```python
from build123d import *

# Parameters (mm, degrees)
SKETCH1_R           = 4.826
BOSS_EXTRUDE1_DEPTH = 9.652
SKETCH2_W           = 57.404
SKETCH2_H           = 3.048
CUT_EXTRUDE1_DEPTH  = 98.666302935
SKETCH5_W           = 60.452
SKETCH5_H           = 47.752
BOSS_EXTRUDE2_DEPTH = 7.874
FILLET1_R           = 7.874
SKETCH7_R           = 3.937
CUT_EXTRUDE2_DEPTH  = 7.874
RIB1_REACH          = 137.874
SKETCH11_WALL_W     = 341.312489082
SKETCH11_WALL_H     = 7.874


with BuildPart() as part:
    # Sketch1 → Boss-Extrude1 (new body)
    with BuildSketch(Plane(origin=(0, 0, 0), x_dir=(1, 0, 0), z_dir=(0, 1, 0))):
        with BuildLine():
            Line((-25.4, 60.325), (25.4, 60.325))
            ThreePointArc((25.4, 60.325), (34.380256121, 56.605256121), (38.1, 47.625))
            Line((38.1, 47.625), (38.1, -47.625))
            ThreePointArc((38.1, -47.625), (34.380256121, -56.605256121), (25.4, -60.325))
            Line((25.4, -60.325), (-25.4, -60.325))
            ThreePointArc((-25.4, -60.325), (-34.380256121, -56.605256121), (-38.1, -47.625))
            Line((-38.1, -47.625), (-38.1, 47.625))
            ThreePointArc((-38.1, 47.625), (-34.380256121, 56.605256121), (-25.4, 60.325))
        make_face()
        with Locations(Location((-25.4, -47.625, 0), (0, 0, 270))):
            Circle(SKETCH1_R, mode=Mode.SUBTRACT)
        with Locations(Location((25.4, -47.625, 0), (0, 0, 270))):
            Circle(SKETCH1_R, mode=Mode.SUBTRACT)
        with Locations(Location((25.4, 47.625, 0), (0, 0, 270))):
            Circle(SKETCH1_R, mode=Mode.SUBTRACT)
        with Locations(Location((-25.4, 47.625, 0), (0, 0, 270))):
            Circle(SKETCH1_R, mode=Mode.SUBTRACT)
    extrude(amount=BOSS_EXTRUDE1_DEPTH)

    # Sketch2 → Cut-Extrude1 (cut, through all)
    with BuildSketch(Plane.ZY.offset(38.1)):
        Rectangle(SKETCH2_W, SKETCH2_H)
    extrude(amount=-CUT_EXTRUDE1_DEPTH, mode=Mode.SUBTRACT)



with BuildPart() as body_2:
    # Sketch5 → Boss-Extrude2 (new body)
    with BuildSketch(Plane(origin=(-42.960508789, 74.409783942, 0), x_dir=(0.8660254037844399, 0.49999999999999795, 0), z_dir=(0.4999999999999979, -0.8660254037844398, 0))):
        with Locations((35.838432116, 0)):
            Rectangle(SKETCH5_W, SKETCH5_H)
    extrude(amount=-BOSS_EXTRUDE2_DEPTH)

    # Fillet1
    fillet1_edges = [body_2.edges().sort_by_distance(p)[0] for p in [
        (-40.0685, 80.625542015, 23.876),
        (12.28446771, 110.851542015, 23.876),
        (12.28446771, 110.851542015, -23.876),
        (-40.0685, 80.625542015, -23.876),
    ]]
    fillet(fillet1_edges, radius=FILLET1_R)

    # Sketch7 → Cut-Extrude2 (cut)
    with BuildSketch(Plane(origin=(-46.897508789, 81.228867971, 0), x_dir=(0.8660254037844398, 0.49999999999999806, 0), z_dir=(-0.499999999999998, 0.8660254037844397, 0))):
        with Locations(Location((13.486432116, 16.002, 0), (0, 0, 180))):
            Circle(SKETCH7_R)
        with Locations(Location((13.486432116, -16.002, 0), (0, 0, 180))):
            Circle(SKETCH7_R)
        with Locations(Location((58.190432116, -16.002, 0), (0, 0, 180))):
            Circle(SKETCH7_R)
        with Locations(Location((58.190432116, 16.002, 0), (0, 0, 180))):
            Circle(SKETCH7_R)
    extrude(amount=-CUT_EXTRUDE2_DEPTH, mode=Mode.SUBTRACT)


with BuildPart() as part_1:
    add(part.part)

    add(body_2.part)  # Loft1 merges body 2
    # Sketch3 → Loft1 section 0
    with BuildSketch(Plane(origin=(0, 9.652, 0), x_dir=(1, 0, 0), z_dir=(0, 1, 0))):
        with BuildLine():
            Line((8.005076562, 60.325), (-7.211701075, 60.325))
            Line((-7.211701075, 60.325), (-7.211701075, -60.325))
            Line((-7.211701075, -60.325), (8.005076562, -60.325))
            Line((8.005076562, -60.325), (8.005076562, 60.325))
        make_face()
    # Sketch10 → Loft1 section 1
    with BuildSketch(Plane(origin=(-42.960508789, 74.409783942, 0), x_dir=(0.8660254037844398, 0.49999999999999806, 0), z_dir=(0.499999999999998, -0.8660254037844397, 0))):
        with BuildLine():
            Line((53.543522628, 23.876), (45.669522628, 23.876))
            Line((45.669522628, 23.876), (45.669522628, -23.876))
            Line((45.669522628, -23.876), (53.543522628, -23.876))
            Line((53.543522628, -23.876), (53.543522628, 23.876))
        make_face()
    loft()

    # Sketch11 wall → Rib1 (add, up to next)
    with BuildSketch(Plane(origin=(-38.1, 43.434, 0), x_dir=(0, 1, 0), z_dir=(-1, 0, 0)), mode=Mode.PRIVATE) as rib1_sk1:
        Rectangle(SKETCH11_WALL_W, SKETCH11_WALL_H)
    rib1_tool1 = extrude(rib1_sk1.sketch, amount=-RIB1_REACH, mode=Mode.PRIVATE) - part_1.part
    add(rib1_tool1.solids().sort_by_distance((-38.1, 43.434, 0))[0])


solid = part_1.part
```
Geometry: final body of the model. Coordinates: model frame, mm. A direction names the side the tool comes from. Round coordinates to 2 decimals unless told otherwise and drop trailing zeros. Loops run counter-clockwise (first coordinate to the right, second up) from the corner with the lowest first, then second, coordinate; pieces in that order, holes last.
Item 1: Section B-B, the plane x = -16. Output: boundary loops of the cut face in (y, z) (3 decimals).
Checked values:
outline: (0, -60.325) - (9.652, -60.325) - (9.652, -3.937) - (89.975, -3.937) - (89.975, -23.876) - (99.068, -23.876) - (99.068, 23.876) - (89.975, 23.876) - (89.975, 3.937) - (9.652, 3.937) - (9.652, 60.325) - (0, 60.325) - (0, 28.702) - (1.524, 28.702) - (1.524, -28.702) - (0, -28.702) - close
Item 2: Mould query, pull axis Z, two halves, no side actions, for faces 4 (the flat face through (1, 0, -45)), 5 (the flat face through (-1, 1.524, 0)), 6 (the cylindrical face through (7.951, 108.413, 18.663)), 7 (the cylindrical face through (34.478, 4.758, 56.506)). Classes: released by +Z, released by -Z, zero draft, split by the parting line, or undercut.
Checked values:
face 4: zero draft
face 5: undercut
face 6: undercut
face 7: released by +Z
Item 3: Line query: L1, parallel to Y at x = -34.5, z = -37; L2, parallel to Z at x = -8.5, y = 30; L3, parallel to Y at x = 22.5, z = 2. Output: solid intervals per line, ascending.
Checked values:
L1: y = 0 to 9.65
L2: z = -3.94 to 3.94
L3: y = 1.52 to 9.65
Item 4: Reachability of faces 1 (the flat face through (-22, 9.652, -33)), 2 (the flat face through (-22, 9.652, 32)), 3 (the flat face through (-21, 53, 3.937)) from +Z, -Z, +X, -X, +Y, -Y: full face, straight path, thin tool, end or side. Return the list, or none.
Checked values:
face 1: -Z, -X
face 2: +Z, -X
face 3: +Z
Item 5: Section A-A, the plane y = 7. Output: boundary loops of the cut face in (x, z) (3 decimals).
Checked values:
outline: (-38.1, -47.625) arc R12.7 ccw to (-25.4, -60.325) - (25.4, -60.325) arc R12.7 ccw to (38.1, -47.625) - (38.1, 47.625) arc R12.7 ccw to (25.4, 60.325) - (-25.4, 60.325) arc R12.7 ccw to (-38.1, 47.625) - close; hole circle Ø9.652 at (-25.4, -47.625); hole circle Ø9.652 at (-25.4, 47.625); hole circle Ø9.652 at (25.4, -47.625); hole circle Ø9.652 at (25.4, 47.625)
Item 6: Contact query for flat-ended pins moving along their axis: P1, Ø1.5, axis at x = 2, z = -1, coming from the -Y side; P2, Ø24, axis at x = 24, z = -28.5, coming from the +Y side; P3, Ø24.5, axis at x = -21, z = -25.5, coming from the +Y side. Output: stop coordinate, or through.
Checked values:
P1: stops at y = 1.52
P2: stops at y = 9.65
P3: stops at y = 103.19
